Read the model definition and answer for the solid it produces. Units are mm, in the model's axes. A direction names the side the tool comes from. Coordinates: 2 decimals unless noted, no trailing zeros. Write each loop counter-clockwise with the first axis right and the second up, starting at its lowest first coordinate (ties: lowest second). Pieces come first, ordered by that corner, then holes.
from build123d import *

# Parameters (mm, degrees)
SKETCH1_W           = 290
SKETCH1_H           = 595
BOSS_EXTRUDE2_DEPTH = 405
FILLET3_R           = 10
SKETCH3_W           = 575
SKETCH3_H           = 385
CUT_EXTRUDE2_DEPTH  = 270


with BuildPart() as part:
    # Sketch1 → Boss-Extrude2 (new body)
    with BuildSketch(Plane(origin=(0, 0, 0), x_dir=(1, 0, 0), z_dir=(0, 1, 0))):
        Rectangle(SKETCH1_W, SKETCH1_H)
    extrude(amount=BOSS_EXTRUDE2_DEPTH)

    # Fillet3
    fillet3_edges = [part.edges().sort_by_distance(p)[0] for p in [
        (0, 405, 297.5),
        (145, 405, 0),
        (0, 0, 297.5),
        (0, 0, -297.5),
        (145, 0, 0),
        (145, 202.5, 297.5),
        (145, 202.5, -297.5),
        (0, 405, -297.5),
    ]]
    fillet(fillet3_edges, radius=FILLET3_R)

    # Sketch3 → Cut-Extrude2 (cut)
    with BuildSketch(Plane.ZY.offset(145)):
        with Locations((0, 202.5)):
            Rectangle(SKETCH3_W, SKETCH3_H)
    extrude(amount=-CUT_EXTRUDE2_DEPTH, mode=Mode.SUBTRACT)


solid = part.part
Item 1: The part is cut by section B-B (z = 22.5). Give the vertices of the cut face in (x, y).
Item 2: Find the intervals of material crossed by probe 1 along Y at (x, z) = (48, 206); probe 2 along Z at (x, y) = (23, 202); probe 3 along X at (y, z) = (58, -143), in increasing order.
Item 3: The part is cut by section A-A (x = -47.5). Give the vertices of the cut face in (y, z).
Item 4: Determine the mould class of faces 1 (the flat face through (-7, 405, -4)), 2 (the flat face through (-12, 200, -287.5)), 3 (the flat face through (-7, 200, -297.5)) for opening direction Y: +Y half, -Y half, draft (parallel to the pull), parting line (faces both ways), or undercut.
Item 5: The part is cut by section C-C (y = 94.5). Give the vertices of the cut face in (x, z).
Item 6: Given pin 1 (2 mm diameter, centred on y = 143.5, z = -170.5, fed in from -X), flat-ended and moving along its own axis, determine where the tip first touches the part or whether it passes through.
Item 7: For faces 4 (the flat face through (-7, 0, -4)), 5 (the flat face through (125, 205, -4)), determine the directions among +Z, -Z, +X, -X, +Y, -Y from which every point of the face is accessible in a straight line to the end or side of a thin tool.
Answer:
1. outline: (-145, 0) - (135, 0) arc R10 ccw to (145, 10) - (145, 395) arc R10 ccw to (135, 405) - (-145, 405) - (-145, 395) - (125, 395) - (125, 10) - (-145, 10) - close
2. probe 1: y = 0 to 10, 395 to 405
2. probe 2: z = -297.5 to -287.5, 287.5 to 297.5
2. probe 3: x = 125 to 145
3. outline: (0, -287.5) arc R10 ccw to (10, -297.5) - (395, -297.5) arc R10 ccw to (405, -287.5) - (405, 287.5) arc R10 ccw to (395, 297.5) - (10, 297.5) arc R10 ccw to (0, 287.5) - close; hole (10, -287.5) - (395, -287.5) - (395, 287.5) - (10, 287.5) - close
4. face 1: +Y half
4. face 2: undercut
4. face 3: draft
5. outline: (-145, -297.5) - (135, -297.5) arc R10 ccw to (145, -287.5) - (145, 287.5) arc R10 ccw to (135, 297.5) - (-145, 297.5) - (-145, 287.5) - (125, 287.5) - (125, -287.5) - (-145, -287.5) - close
6. pin 1: stops at x = 125
7. face 4: +Z, -Z, +X, -X, -Y
7. face 5: -X
